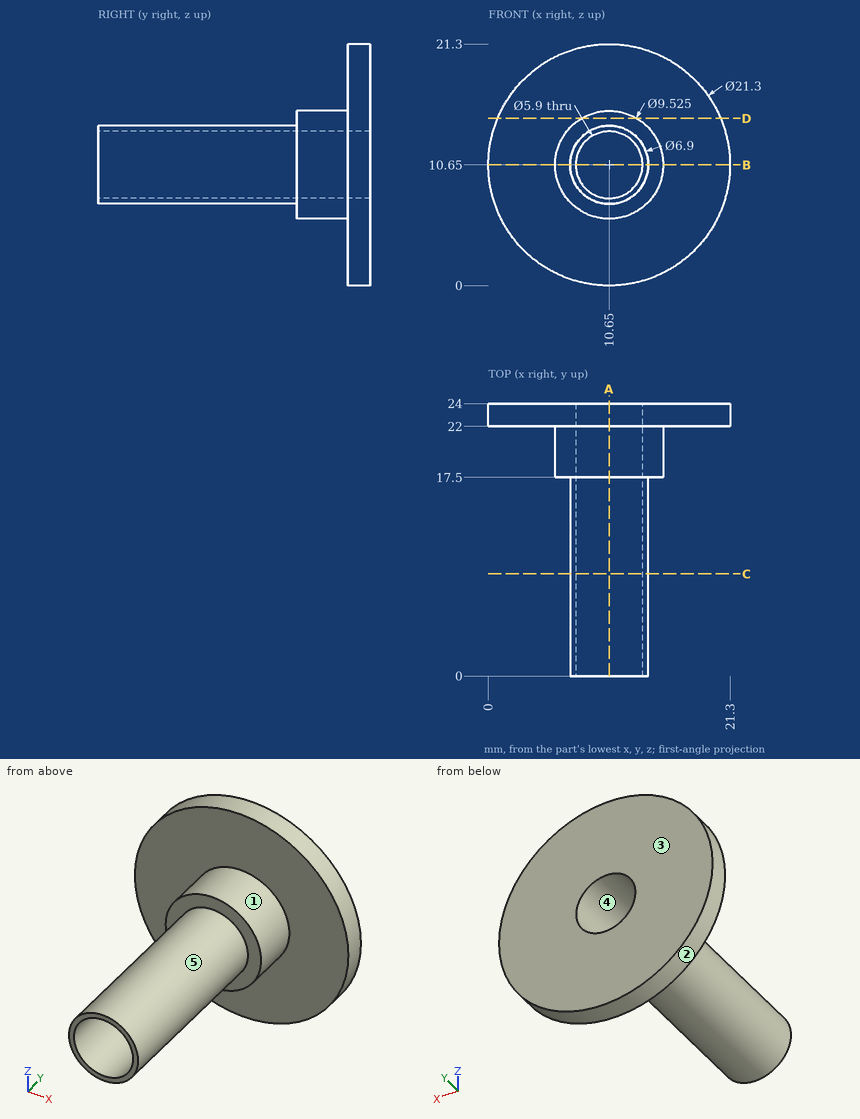
Design review of the part shown in the three views and the two pictorial views. Dimensions are in mm from the part's minimum x, y and z. A direction names the side the tool comes from. Round coordinates to 2 decimals unless told otherwise and drop trailing zeros. Write each loop counter-clockwise with the first axis right and the second up, starting at its lowest first coordinate (ties: lowest second). Pieces come first, ordered by that corner, then holes. Notation, with made-up numbers: M 31,-16 L 63,-16 A23 ccw 63,-7 Z; hole C -24.75,26 d1. An arc over 180 degrees is marked long. One line per item, written item: value. Start each with the question number.
1. Take a section at D-D on z = 14.75. State the section outline as (x, y) points, then the cut area to 3 significant figures.
2. Take a section at A-A on x = 10.65. State the section outline as (y, z) points.
3. To check wall thickness, follow probe 1 along Z at (x, y) = (10.65, 11.75); probe 2 along Z at (x, y) = (10.65, 18.5); probe 3 along X at (y, z) = (12.5, 9.75). State the ranges of each line that lie inside material, in increasing order. Write a range as from..to.
4. Clearance check with flat-ended pins moving along their axes: P1, Ø12, axis at y = 13, z = 4, coming from the +X side; P2, Ø8, axis at y = 2.5, z = 14.5, coming from the -X side; P3, Ø8, axis at y = 11, z = 17, coming from the -X side; P4, Ø2, axis at x = 3, y = 18, coming from the +Z side. State where each tip first meets the part, or that it passes through.
5. Take a section at C-C on y = 9. State the section outline as (x, z) points.
6. For the marked faces 1 and 2, list the 3-axis set-ups (+Z, -Z, +X, -X, +Y, -Y) from which the entire face can be reached by the end or side of a thin tool; tool diameter is ignored.
7. Draft analysis for pull direction X (two halves, no side actions). For the marked faces 3, 4 and 5, state which applies: pulls with the +X half, pulls with the -X half, needs draft (parallel to the pull), parting line crosses it, or undercut.
8. Take a section at B-B on z = 10.65. State the section outline as (x, y) points.
Computed:
1. outline: M 0.82,22 L 8.23,22 L 8.23,17.5 L 13.07,17.5 L 13.07,22 L 20.48,22 L 20.48,24 L 0.82,24 Z
1. area: 61.1 mm²
2. outline: M 0,7.2 L 17.5,7.2 L 17.5,5.89 L 22,5.89 L 22,0 L 24,0 L 24,7.7 L 0,7.7 Z; M 0,13.6 L 24,13.6 L 24,21.3 L 22,21.3 L 22,15.41 L 17.5,15.41 L 17.5,14.1 L 0,14.1 Z
3. probe 1: z = 7.2..7.7, 13.6..14.1
3. probe 2: z = 5.89..7.7, 13.6..15.41
3. probe 3: x = 7.32..7.84, 13.46..13.98
4. P1: stops at x = 14.59
4. P2: stops at x = 7.2
4. P3: stops at x = 8.12
4. P4: passes through
5. outline: C 10.65,10.65 d6.9; hole C 10.65,10.65 d5.9
6. face 1: -Y
6. face 2: +Y, -Y
7. face 3: needs draft
7. face 4: undercut
7. face 5: parting line crosses it
8. outline: M 0,22 L 5.89,22 L 5.89,17.5 L 7.2,17.5 L 7.2,0 L 7.7,0 L 7.7,24 L 0,24 Z; M 13.6,0 L 14.1,0 L 14.1,17.5 L 15.41,17.5 L 15.41,22 L 21.3,22 L 21.3,24 L 13.6,24 Z
